Verification items for the finished model (mm, model axes). Give positions to 0.01 mm unless a question says otherwise; leave off trailing zeros. Loops run counter-clockwise (first coordinate to the right, second up) from the corner with the lowest first, then second, coordinate; pieces in that order, holes last. Notation, with made-up numbers: (81, 66) - (140, 66) arc R25 ccw to (140, 79) - close; hole circle Ø10 at (62.5, 50.5). An arc over 180 degrees is marked (long way). Use one line per item in the form item = value.
```python
from build123d import *

# Parameters (mm, degrees)
SKETCH_1_R          = 47
SKETCH_1_R_2        = 1.7
SKETCH_1_W          = 40.5
SKETCH_1_H          = 20
EXTRUDE_1_DEPTH     = 5
CUT_EXTRUDE_1_DEPTH = 2
CUT_EXTRUDE_2_DEPTH = 1
CUT_EXTRUDE_3_DEPTH = 6
FILLET_1_R          = 2


with BuildPart() as part:
    # Эскиз1 → Бобышка-Вытянуть1 (new body)
    with BuildSketch(Plane(origin=(0, 0, 0), x_dir=(1, 0, 0), z_dir=(0, 1, 0))):
        Circle(SKETCH_1_R)
        with Locations((-15, 5)):
            Circle(SKETCH_1_R_2, mode=Mode.SUBTRACT)
        with Locations((-15, -5)):
            Circle(SKETCH_1_R_2, mode=Mode.SUBTRACT)
        with Locations((36, 5)):
            Circle(SKETCH_1_R_2, mode=Mode.SUBTRACT)
        with Locations((36, -5)):
            Circle(SKETCH_1_R_2, mode=Mode.SUBTRACT)
        with Locations((10.5, 0)):
            Rectangle(SKETCH_1_W, SKETCH_1_H, mode=Mode.SUBTRACT)
    extrude(amount=EXTRUDE_1_DEPTH)

    # Эскиз2 → Вырез-Вытянуть1 (cut)
    with BuildSketch(Plane(origin=(0, 5, 0), x_dir=(1, 0, 0), z_dir=(0, 1, 0))):
        Polygon((-12, 6.732050808), (-15, 8.464101615), (-18, 6.732050808), (-18, 3.267949192), (-15, 1.535898385), (-12, 3.267949192), align=None)
        Polygon((-12, -3.267949192), (-15, -1.535898385), (-18, -3.267949192), (-18, -6.732050808), (-15, -8.464101615), (-12, -6.732050808), align=None)
        Polygon((36, 8.464101615), (33, 6.732050808), (33, 3.267949192), (36, 1.535898385), (39, 3.267949192), (39, 6.732050808), align=None)
        Polygon((36, -1.535898385), (33, -3.267949192), (33, -6.732050808), (36, -8.464101615), (39, -6.732050808), (39, -3.267949192), align=None)
    extrude(amount=-CUT_EXTRUDE_1_DEPTH, mode=Mode.SUBTRACT)

    # Эскиз3 → Вырез-Вытянуть2 (cut, symmetric)
    with BuildSketch(Plane.XY):
        Polygon((27.412104095, 3.670718329), (30.75, 0), (38.308934037, 0), align=None)
        Polygon((-6.412104095, 3.670718329), (-9.75, 0), (-17.308934037, 0), align=None)
    extrude(amount=CUT_EXTRUDE_2_DEPTH, both=True, mode=Mode.SUBTRACT)

    # Эскиз4 → Вырез-Вытянуть3 (cut, through all)
    with BuildSketch(Plane(origin=(0, 5, 0), x_dir=(1, 0, 0), z_dir=(0, 1, 0))):
        with BuildLine():
            ThreePointArc((-38.832975678, -16), (0, -42), (38.832975678, -16))
            Line((38.832975678, -16), (-38.832975678, -16))
        make_face()
        with BuildLine():
            ThreePointArc((38.832975678, 16), (0, 42), (-38.832975678, 16))
            Line((-38.832975678, 16), (38.832975678, 16))
        make_face()
        with BuildLine():
            Line((-35.623026261, -10), (-20.75, -10))
            Line((-20.75, -10), (-20.75, 10))
            Line((-20.75, 10), (-35.623026261, 10))
            ThreePointArc((-35.623026261, 10), (-37, 0), (-35.623026261, -10))
        make_face()
    extrude(amount=-CUT_EXTRUDE_3_DEPTH, mode=Mode.SUBTRACT)

    # Скругление1
    fillet_1_edges = [part.edges().sort_by_distance(p)[0] for p in [
        (-38.832975678, 2.5, 16),
        (38.832975678, 2.5, 16),
        (38.832975678, 2.5, -16),
        (-38.832975678, 2.5, -16),
    ]]
    fillet(fillet_1_edges, radius=FILLET_1_R)


solid = part.part
```
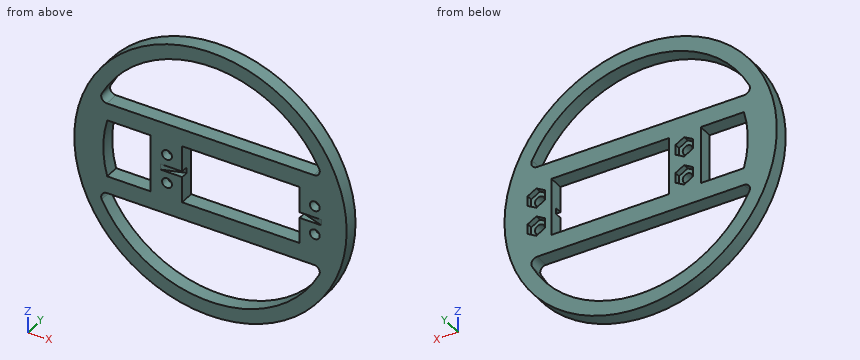
1. Section check C-C, the plane x = 22.5. Record the cut outline in (y, z).
Result set:
outline = (0, -41.26) - (5, -41.26) - (5, -35.46) - (0, -35.46) - close; (0, -16) - (5, -16) - (5, -10) - (0, -10) - close; (0, 10) - (5, 10) - (5, 16) - (0, 16) - close; (0, 35.46) - (5, 35.46) - (5, 41.26) - (0, 41.26) - close
2. Depth check by flat-ended pin: pin 1 Ø2.5 at (x, y) = (-17.5, 3.5) entering from +Z; pin 2 Ø2 at (y, z) = (4, 5) entering from +X; pin 3 Ø3 at (x, y) = (35, 1) entering from +Z. Enter the tip coordinate at first touch or a pass-through.
Result set:
pin_1 = 44.1
pin_2 = 46.83
pin_3 = 32.97
3. Section check A-A, the plane x = 0. Record the cut outline in (y, z), then the cut area to 3 significant figures.
Result set:
outline = (0, -47) - (5, -47) - (5, -42) - (0, -42) - close; (0, -16) - (5, -16) - (5, -10) - (0, -10) - close; (0, 10) - (5, 10) - (5, 16) - (0, 16) - close; (0, 42) - (5, 42) - (5, 47) - (0, 47) - close
area = 110 mm²
4. Scan lines: probe 1 along X at (y, z) = (0.85, 9); probe 2 along Z at (x, y) = (-27, 0.8); probe 3 along X at (y, z) = (1.15, 2.5). Record each from-to range of solid material in increasing order.
Result set:
probe_1 = -46.13 to -35.89, -20.75 to -9.75, 30.75 to 46.13
probe_2 = -38.47 to -32.17, -16 to -10, 10 to 16, 32.17 to 38.47
probe_3 = -46.93 to -36.92, -20.75 to -9.75, 30.75 to 46.93
5. Section check B-B, the plane z = 5. Record the cut outline in (x, y).
Result set:
outline = (-46.73, 0) - (-36.66, 0) - (-36.66, 5) - (-46.73, 5) - close; (-20.75, 0) - (-16.7, 0) - (-16.7, 3) - (-18, 3) - (-18, 5) - (-20.75, 5) - close; (-13.3, 0) - (-9.75, 0) - (-9.75, 5) - (-12, 5) - (-12, 3) - (-13.3, 3) - close; (30.75, 0) - (34.3, 0) - (34.3, 3) - (33, 3) - (33, 5) - (30.75, 5) - close; (37.7, 0) - (46.73, 0) - (46.73, 5) - (39, 5) - (39, 3) - (37.7, 3) - close
6. Section check D-D, the plane x = -41. Record the cut outline in (y, z).
Result set:
outline = (0, -22.98) - (5, -22.98) - (5, 22.98) - (0, 22.98) - close
